Part model, mm, in its own coordinate system. Face numbers are marked on the shaded views. A direction names the side the tool comes from. Coordinates: 2 decimals unless noted, no trailing zeros. Write each loop counter-clockwise with the first axis right and the second up, starting at its lowest first coordinate (ties: lowest second). Pieces come first, ordered by that corner, then holes. Notation, with made-up numbers: (23, 25.5) -> (70, 25.5) arc R17 ccw to (70, 33.5) -> close; hole circle Ø8 at (-32.75, 58.25). An arc over 180 degrees is marked (long way). One line per question, with ' | ' between items. Start each with the question number.
Item 1: Saw through at C-C (y = 13.75). List the corners of the cut face in (x, z).
Item 2: Saw through at A-A (y = 0). List the corners of the cut face in (x, z).
Item 3: 3-axis set-ups, long thin cutter, end or side, ignore diameter. For the marked faces 5 and 6: which of +Z, -Z, +X, -X, +Y, -Y reach the whole face in a straight line?
Item 4: Probe probe 1 along Y at (x, z) = (1, 1); probe 2 along Y at (x, z) = (23, 2.25); probe 3 along Y at (x, z) = (-19.5, 2). List the from-to ranges inside material, lowest first. Write a range as [from, to].
Item 5: Saw through at B-B (x = 0). List the corners of the cut face in (y, z), and give its area (3 significant figures).
Item 6: Pin check, flat tips, straight feed: pin 1 (3.5 mm diameter, centred on x = -23.82, y = 13.75, fed in from +Z); pin 2 (4.5 mm diameter, centred on x = 0.5, y = -1, fed in from -Z); pin 3 (19.5 mm diameter, centred on x = -6.5, y = 1, fed in from -Z); pin 4 (3 mm diameter, centred on x = -14, z = 2, fed in from +Y). Stop position of each tip, or through.
Item 7: Two-plate mould, pull along Y, no slides. Class the marked faces 1, 2, 3 and 4: pulls with the +Y half, pulls with the -Y half, needs draft (parallel to the pull), parting line crosses it, or undercut.
Item 8: Saw through at D-D (x = 18.5). List the corners of the cut face in (y, z), and give its area (3 significant figures).
from build123d import *

# Parameters (mm, degrees)
SKETCH1_R           = 2.1
BOSS_EXTRUDE1_DEPTH = 7
BOSS_EXTRUDE2_START = 2
BOSS_EXTRUDE2_DEPTH = 2
SKETCH3_R           = 7.05
CUT_EXTRUDE1_DEPTH  = 5
SKETCH4_R           = 7.5
CUT_EXTRUDE2_DEPTH  = 2


with BuildPart() as part:
    # Sketch1 → Boss-Extrude1 (new body)
    with BuildSketch(Plane.XY):
        with BuildLine():
            Line((-28.559544782, -15.511363636), (-21.718978566, -28.10622388))
            ThreePointArc((-21.718978566, -28.10622388), (-23.583461057, -35.132547662), (-16.46241644, -36.594137349))
            ThreePointArc((-16.46241644, -36.594137349), (0, -44), (16.46241644, -36.594137349))
            ThreePointArc((16.46241644, -36.594137349), (23.583461057, -35.132547662), (21.718978566, -28.10622388))
            Line((21.718978566, -28.10622388), (28.559544782, -15.511363636))
            ThreePointArc((28.559544782, -15.511363636), (0, 32.5), (-28.559544782, -15.511363636))
        make_face()
        with Locations((-23.815698604, 13.75)):
            Circle(SKETCH1_R, mode=Mode.SUBTRACT)
        with Locations((23.815698604, 13.75)):
            Circle(SKETCH1_R, mode=Mode.SUBTRACT)
        with Locations((-19.332614929, -32.5)):
            Circle(SKETCH1_R, mode=Mode.SUBTRACT)
        with Locations((19.332614929, -32.5)):
            Circle(SKETCH1_R, mode=Mode.SUBTRACT)
    extrude(amount=BOSS_EXTRUDE1_DEPTH)

    # Sketch2 → Boss-Extrude2 (add)
    with BuildSketch(Plane(origin=(0, 0, 0), x_dir=(-1, 0, 0), z_dir=(0, 0, -1)).offset(BOSS_EXTRUDE2_START)):
        with BuildLine():
            Line((-23.726391049, -12.886363636), (-14.499461197, -29.875))
            ThreePointArc((-14.499461197, -29.875), (0, -38.5), (14.499461197, -29.875))
            Line((14.499461197, -29.875), (23.726391049, -12.886363636))
            ThreePointArc((23.726391049, -12.886363636), (26.991956985, -0.65898263), (24.326965388, 11.713187226))
            ThreePointArc((24.326965388, 11.713187226), (21.997045256, 12.7), (22.307400391, 15.21117641))
            ThreePointArc((22.307400391, 15.21117641), (0, 27), (-22.307400391, 15.21117641))
            ThreePointArc((-22.307400391, 15.21117641), (-21.997045256, 12.7), (-24.326965388, 11.713187226))
            ThreePointArc((-24.326965388, 11.713187226), (-26.991956985, -0.65898263), (-23.726391049, -12.886363636))
        make_face()
        with BuildLine():
            Line((-21.090125377, -11.454545455), (-11.863195525, -28.443181818))
            ThreePointArc((-11.863195525, -28.443181818), (0, -35.5), (11.863195525, -28.443181818))
            Line((11.863195525, -28.443181818), (21.090125377, -11.454545455))
            ThreePointArc((21.090125377, -11.454545455), (0, 24), (-21.090125377, -11.454545455))
        make_face(mode=Mode.SUBTRACT)
    extrude(amount=-BOSS_EXTRUDE2_DEPTH)

    # Sketch3 → Cut-Extrude1 (cut)
    with BuildSketch(Plane(origin=(0, 0, 0), x_dir=(-1, 0, 0), z_dir=(0, 0, -1))):
        with Locations((0, -22)):
            Circle(SKETCH3_R)
    extrude(amount=-CUT_EXTRUDE1_DEPTH, mode=Mode.SUBTRACT)

    # Sketch4 → Cut-Extrude2 (cut)
    with BuildSketch(Plane(origin=(0, 0, 0), x_dir=(-1, 0, 0), z_dir=(0, 0, -1))):
        Circle(SKETCH4_R)
    extrude(amount=-CUT_EXTRUDE2_DEPTH, mode=Mode.SUBTRACT)


solid = part.part
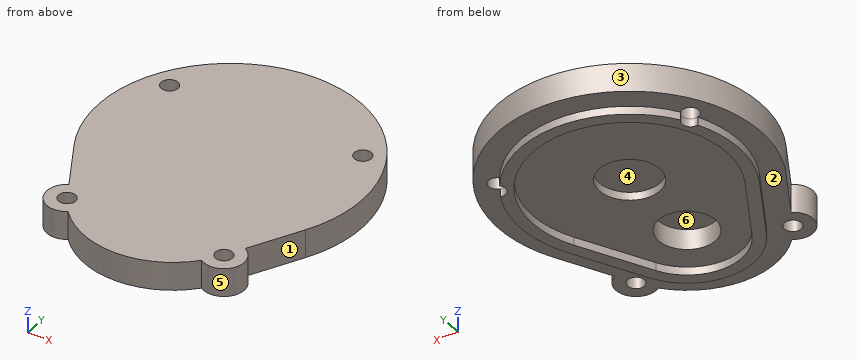
From the geometry:
1) outline: (-29.45, 0) -> (-25.92, 0) -> (-25.92, 7) -> (-29.45, 7) -> close; (-21.72, -2) -> (-19.67, -2) -> (-19.67, 0) -> (19.67, 0) -> (19.67, -2) -> (21.72, -2) -> (21.72, 7) -> (-21.72, 7) -> close; (25.92, 0) -> (29.45, 0) -> (29.45, 7) -> (25.92, 7) -> close
2) outline: (-32.5, 0) -> (-27, 0) -> (-27, -2) -> (-24, -2) -> (-24, 0) -> (-7.5, 0) -> (-7.5, 2) -> (7.5, 2) -> (7.5, 0) -> (24, 0) -> (24, -2) -> (27, -2) -> (27, 0) -> (32.5, 0) -> (32.5, 7) -> (-32.5, 7) -> close
3) face 5: +Z, -Z | face 6: -Z
4) probe 1: [-43.98, -28.98], [-15.02, -7.43], [7.43, 32.48] | probe 2: [-35.9, -29.1], [-25.75, 11.81], [15.69, 22.96] | probe 3: [-37.5, -34.59], [-30.41, 26]
5) outline: (-44, 0) -> (-38.5, 0) -> (-38.5, -2) -> (-35.5, -2) -> (-35.5, 0) -> (-29.05, 0) -> (-29.05, 5) -> (-14.95, 5) -> (-14.95, 0) -> (-7.5, 0) -> (-7.5, 2) -> (7.5, 2) -> (7.5, 0) -> (24, 0) -> (24, -2) -> (27, -2) -> (27, 0) -> (32.5, 0) -> (32.5, 7) -> (-44, 7) -> close | area: 447 mm2
6) pin 1: through | pin 2: z = 2 | pin 3: z = 0 | pin 4: y = 30
7) face 1: undercut | face 2: needs draft | face 3: parting line crosses it | face 4: undercut
8) outline: (-37.43, 0) -> (-34.43, 0) -> (-34.43, 7) -> (-37.43, 7) -> close; (-30.57, 0) -> (-22.51, 0) -> (-22.51, -2) -> (-16.22, -2) -> (-16.22, 0) -> (15.29, 0) -> (15.29, -2) -> (19.67, -2) -> (19.67, 0) -> (26.72, 0) -> (26.72, 7) -> (-30.57, 7) -> close | area: 443 mm2
